```python
from build123d import *

# Parameters (mm, degrees)
F0_R     = 7.62
F1_DEPTH = 17.78
F2_SIZE2 = 9.4794090512
F2_SIZE  = 2.54
F3_R     = 2.54
F4_R     = 3.3655
F5_DEPTH = 12.7


with BuildPart() as f1:
    # F0 (on Top) → F1 (new body)
    with BuildSketch(Plane.XY):
        Circle(F0_R)
    extrude(amount=F1_DEPTH)

    # F2
    f2_edges = [f1.edges().sort_by_distance(p)[0] for p in [
        (-7.62, 0, 17.78),
    ]]
    f2_side = f1.faces().sort_by_distance((0, 0, 17.78))[0]
    chamfer(f2_edges, length=F2_SIZE, length2=F2_SIZE2, reference=f2_side)

    # F3
    f3_edges = [f1.edges().sort_by_distance(p)[0] for p in [
        (-5.08, 0, 17.78),
        (-7.62, 0, 8.300591),
    ]]
    fillet(f3_edges, radius=F3_R)

    # F4 (on face) → F5 (join)
    with BuildSketch(Plane(origin=(0, 0, 0), x_dir=(1, 0, 0), z_dir=(0, 0, -1))):
        Circle(F4_R)
    extrude(amount=F5_DEPTH)


solid = f1.part
```
Could you check a few things on this model? Use its own coordinates, in mm. A direction names the side the tool comes from. Round coordinates to 2 decimals unless told otherwise and drop trailing zeros. Write each loop counter-clockwise with the first axis right and the second up, starting at its lowest first coordinate (ties: lowest second). Pieces come first, ordered by that corner, then holes. Notation, with made-up numbers: M 41,-17.5 L 73,-17.5 A10 ccw 73,-2.5 Z; hole C 54,-27.5 d4. An arc over 180 degrees is marked long. Answer in a Markdown table with one row per item. Add a question column.
Q1. On a 3-axis mill with a long thin cutter (end or side, diameter ignored), from which of +Z, -Z, +X, -X, +Y, -Y can I reach the whole of each face in a straight line? I mean faces 1 (the cylindrical face through (7.268, 2.289, 3.927)), 2 (the flat face through (3, -2, 0)). Say none if no direction works.
Q2. If I drill on line 1 (Y direction, x = -3.25, z = 7); line 2 (X direction, y = 0.25, z = -2.5); line 3 (Y direction, x = 1, z = 11), over which ranges is the centre line in solid material (lowest first)? Write a range as from..to.
Q3. Imagine slicing it at B-B (z = -2). Please give me the cut outline in (x, y), then the cut area to 3 significant figures.
Q4. Will these pins go through, and if not, where does the flat tip stop? pin 1 Ø1 at (y, z) = (3, -3.5) entering from +X; pin 2 Ø1 at (y, z) = (1, 14.5) entering from +X; pin 3 Ø5 at (y, z) = (1.5, -8.5) entering from -X.
Q5. Imagine slicing it at A-A (z = 1.5). Please give me the cut outline in (x, y).
Values:
| question | item | result |
|---|---|---|
| 1 | face 1 | +Z, -Z |
| 1 | face 2 | -Z |
| 2 | line 1 | -6.89..6.89 |
| 2 | line 2 | -3.36..3.36 |
| 2 | line 3 | -6.82..6.82 |
| 3 | outline | C 0,0 d6.73 |
| 3 | area | 35.6 mm^2 |
| 4 | pin 1 | x = 2.25 |
| 4 | pin 2 | x = 6.03 |
| 4 | pin 3 | x = -3.37 |
| 5 | outline | C 0,0 d15.24 |
